from build123d import *

# Parameters (mm, degrees)
BOSS_EXTRUDE1_DEPTH = 14
SKETCH2_W           = 1.5
SKETCH2_H           = 6
CUT_EXTRUDE1_DEPTH  = 22
SKETCH12_W          = 14
SKETCH12_H          = 14
SKETCH12_W_2        = 10.30277124
SKETCH12_H_2        = 10.30277124
CUT_EXTRUDE2_DEPTH  = 18.146428199


with BuildPart() as part:
    # Sketch1 → Boss-Extrude1 (new body)
    with BuildSketch(Plane.XY):
        Polygon((-7, 0), (7, 0), (7, 7), (6.2, 7), (6.2, 1), (3.7, 1), (3.7, 7), (2.9, 7), (2.9, 1), (0.4, 1), (0.4, 7), (-0.4, 7), (-0.4, 1), (-2.9, 1), (-2.9, 7), (-3.7, 7), (-3.7, 1), (-6.2, 1), (-6.2, 7), (-7, 7), align=None)
    extrude(amount=BOSS_EXTRUDE1_DEPTH)

    # Sketch2 → Cut-Extrude1 (cut, through all)
    with BuildSketch(Plane.ZY.offset(7)):
        with Locations((3.125, 4)):
            Rectangle(SKETCH2_W, SKETCH2_H)
        with Locations((7, 4)):
            Rectangle(SKETCH2_W, SKETCH2_H)
        with Locations((10.875, 4)):
            Rectangle(SKETCH2_W, SKETCH2_H)
    extrude(amount=-CUT_EXTRUDE1_DEPTH, mode=Mode.SUBTRACT)

    # Sketch12 → Cut-Extrude2 (cut, through all)
    with BuildSketch(Plane.XZ):
        with Locations((0, 7)):
            Rectangle(SKETCH12_W, SKETCH12_H)
        with Locations((0, 7)):
            Rectangle(SKETCH12_W_2, SKETCH12_H_2, mode=Mode.SUBTRACT)
    extrude(amount=-CUT_EXTRUDE2_DEPTH, mode=Mode.SUBTRACT)


solid = part.part
CAD build for the part. Positions are in the model's coordinates, mm. A direction names the side the tool comes from. Coordinates: 2 decimals unless noted, no trailing zeros. Loops run counter-clockwise (first coordinate to the right, second up) from the corner with the lowest first, then second, coordinate; pieces in that order, holes last. Notation, with made-up numbers: (-36.5, -18) -> (9.5, -18) arc R29 cw to (9.5, 14) -> close; hole circle Ø2 at (3.25, -21). An arc over 180 degrees is marked (long way). One line per item, written item: value.
1. Drill centre lines: line 1 (X direction, y = 4, z = 8); line 2 (Z direction, x = -3.5, y = 2.25) (3 decimals); line 3 (Y direction, x = 4.25, z = 6.5). Where is each one in solid material? Low to high. Write a range as [from, to].
Answers:
line 1: x = [-3.7, -2.9], [-0.4, 0.4], [2.9, 3.7]
line 2: z = [1.849, 2.375], [3.875, 6.25], [7.75, 10.125], [11.625, 12.151]
line 3: y = [0, 1]
2. Slice it at A-A on x = 3.5. Write the cut outline in (y, z) (3 decimals), and give its area (3 significant figures).
Answers:
outline: (0, 1.849) -> (7, 1.849) -> (7, 2.375) -> (1, 2.375) -> (1, 3.875) -> (7, 3.875) -> (7, 6.25) -> (1, 6.25) -> (1, 7.75) -> (7, 7.75) -> (7, 10.125) -> (1, 10.125) -> (1, 11.625) -> (7, 11.625) -> (7, 12.151) -> (0, 12.151) -> close
area: 45.1 mm^2
3. Slice it at B-B on z = 4.25. Write the cut outline in (x, y), and give its area (3 significant figures).
Answers:
outline: (-5.15, 0) -> (5.15, 0) -> (5.15, 1) -> (3.7, 1) -> (3.7, 7) -> (2.9, 7) -> (2.9, 1) -> (0.4, 1) -> (0.4, 7) -> (-0.4, 7) -> (-0.4, 1) -> (-2.9, 1) -> (-2.9, 7) -> (-3.7, 7) -> (-3.7, 1) -> (-5.15, 1) -> close
area: 24.7 mm^2
4. Slice it at D-D on x = 1.5. Write the cut outline in (y, z).
Answers:
outline: (0, 1.85) -> (1, 1.85) -> (1, 12.15) -> (0, 12.15) -> close
5. Which spindle directions (+Z, -Z, +X, -X, +Y, -Y) get a long thin tool onto all of the face, cutting with end or side? Do faces 1 (the face through (3.7, 4, 9)), 2 (the face through (-5.151, 0.5, 6.9)), 3 (the face through (-3.3, 7, 8.9)), 4 (the face through (2.9, 4, 9)), 5 (the face through (0, 4, 2.375)). Say none if no direction does.
Answers:
face 1: +Z, -Z, +X, +Y
face 2: +Z, -Z, -X, +Y, -Y
face 3: +Z, -Z, +X, -X, +Y
face 4: +Z, -Z, +Y
face 5: +X, -X, +Y
6. Pull direction Z, two halves, no side cores. Call faces 6 (the face through (0, 4, 11.625)), 7 (the face through (5.151, 0.5, 6.9)): pulls with the +Z half, pulls with the -Z half, needs draft (parallel to the pull), parting line crosses it, or undercut.
Answers:
face 6: undercut
face 7: needs draft
7. Slice it at C-C on y = 1.75. Give the number of separate pieces and of enclosed holes in the cut face, and give its area (3 significant figures).
Answers:
separate pieces: 12
enclosed holes: 0
area: 13.9 mm^2
8. Flat gauge pins, fed straight in: P1, Ø0.6, axis at y = 3.5, z = 12, coming from the +X side; P2, Ø1.2, axis at y = 5.5, z = 4.5, coming from the -X side. Where does each tip first touch, or does it go through?
Answers:
P1: stops at x = 3.7
P2: stops at x = -3.7
